Autodesk Inventor part; units mm, degrees
ref_plane "YZ Plane" through (0, 0, 0) normal (1, 0, 0) x (0, 1, 0)
ref_plane "XZ Plane" through (0, 0, 0) normal (0, 1, 0) x (-1, 0, 0)
ref_plane "XY Plane" through (0, 0, 0) normal (0, 0, 1) x (1, 0, 0)
sketch "Boceto1" plane through (0, 0, 0) normal (0, 1, 0) x (-1, 0, 0)
  circle A0 centre (0, 0) radius 20
  circle A1 centre (0, 0) radius 30
  line L0 (0, 0) -> (0, 60)
  line L1 (0, 60) -> (5, 60)
  line L2 (5, 60) -> (-5, 60)
  line L3 (-5, 60) -> (-5, 0)
  line L4 (-5, 0) -> (5, 0)
  line L5 (5, 0) -> (5, 60)
  line L6 (0, 60) -> (30, 60)
  line L7 (30, 60) -> (-30, 60)
  line L8 (-30, 60) -> (-30, 75)
  line L9 (-30, 75) -> (30, 75)
  line L10 (30, 75) -> (30, 60)
  point P0 (-5, 29.5804)
  point P1 (5, 29.5804)
  dimension "d0" = 40
  dimension "d1" = 60
  dimension "d2" = 60
  dimension "d3" = 5
  dimension "d4" = 10
  dimension "d5" = 30
  dimension "d6" = 60
  dimension "d7" = 15
extrude "Extrusión1" add sketch "Boceto1" along normal blind 60
sketch "Boceto2" plane through (30, 0, 75) normal (1, 0, 0) x (0, 0, -1)
  line L0 (0, 60) -> (15, 60)
  line L1 (0, 60) -> (0, 15)
  line L2 (0, 0) -> (0, 60)
  line L3 (0, 15) -> (75, 15)
  line L4 (75, 15) -> (75, 30)
  line L5 (75, 30) -> (15, 30)
  line L6 (15, 0) -> (15, 60)
  point P0 (75, 0)
  point P1 (15, 15)
  dimension "d10" = 45
  dimension "d11" = 15
extrude "Extrusión2" add sketch "Boceto2" against normal blind 60 contours L5 L4 L3 L6
sketch "Boceto3" plane through (30, 0, 75) normal (1, 0, 0) x (0, 0, -1)
  line L0 (45.4196, 15) -> (15, 15)
  line L1 (15, 15) -> (0, 15)
  line L2 (0, 0) -> (0, 60)
  line L3 (45.4196, 0) -> (15, 0)
  line L4 (0, 15) -> (45.4196, 15)
  line L5 (45.4196, 15) -> (45.4196, 0)
  line L6 (45.4196, 0) -> (0, 0)
  line L7 (0, 0) -> (0, 15)
  point P0 (75, 0)
extrude "Extrusión3" cut sketch "Boceto3" against normal blind 60
sketch "Boceto4" plane through (-30, 60, 75) normal (0, 0, 1) x (1, 0, 0)
  line L0 (60, 0) -> (0, 0)
  line L1 (30, 0) -> (47.5, 0)
  line L2 (47.5, 0) -> (47.5, -15)
  line L3 (30, 0) -> (30, -5.3607)
  circle A0 centre (47.5, -15) radius 8
  circle A1 centre (12.5, -15) radius 8
  point P0 (30, -60)
  point P1 (35, 0)
  point P2 (25, 0)
  dimension "d16" = 17.5
  dimension "d17" = 15
  dimension "d18" = 16
extrude "Extrusión4" cut sketch "Boceto4" against normal blind 15
sketch "Boceto5" plane through (0, 60, 0) normal (0, 1, 0) x (1, 0, 0)
  circle A0 centre (0, 0) radius 20
  dimension "d21" = 40
extrude "Extrusión5" cut sketch "Boceto5" against normal blind 60
sketch "Boceto6" plane through (0, 0, 0) normal (0, -1, 0) x (1, 0, 0)
  line L0 (0, 0) -> (0, -75)
  circle A0 centre (0, -75) radius 10
  circle A1 centre (0, -75) radius 23
  line L1 (0, -75) -> (23, -75)
  arc A2 (-5, 29.5804) -> (5, 29.5804) centre (0, 0) ccw
  line L2 (23, -19.2614) -> (23, -75)
  line L3 (-23, -19.2614) -> (-23, -75)
  dimension "d24" = 75
  dimension "d25" = 20
  dimension "d26" = 46
extrude "Extrusión6" add sketch "Boceto6" against normal blind 15 contours A2 L2 A1 L0 | L0 A1 L3 A2 | A1 L1 A0 L0 | L0 A0 L1 A1
sketch "Boceto7" plane through (0, 60, 0) normal (0, 1, 0) x (1, 0, 0)
  arc A0 (5, -29.5804) -> (-5, -29.5804) centre (0, 0) ccw
  line L0 (0, 30) -> (0, 55)
  line L1 (0, 55) -> (5, 55)
  line L2 (5, 29.5804) -> (5, 55)
  line L3 (0, 55) -> (-5, 55)
  line L4 (-5, 29.5804) -> (-5, 55)
  arc A1 (5, 29.5804) -> (-5, 29.5804) centre (0, 0) ccw
  dimension "d29" = 25
  dimension "d30" = 5
extrude "Extrusión7" add sketch "Boceto7" against normal blind 45
sketch "Boceto8" plane through (-5, 60, -55) normal (-1, 0, 0) x (0, 0, 1)
  line L0 (0, 0) -> (0, -45)
  line L1 (84.5804, 0) -> (25.4196, 0)
  line L2 (0, -45) -> (25.4196, 0)
  line L3 (35.7386, -45) -> (25.4196, -45)
  line L4 (25.4196, 0) -> (25.4196, -45)
  line L5 (25.4196, -45) -> (0, -45)
  line L6 (0, -45) -> (0, 0)
  line L7 (25.4196, 0) -> (0, 0)
  point P0 (55, -60)
extrude "Extrusión8" cut sketch "Boceto8" against normal blind 45 contours L7 L2 L0
Geometry check sheet. Reference: the model listing, model coordinates, mm. A direction names the side the tool comes from. Round coordinates to 2 decimals unless told otherwise and drop trailing zeros. Loops run counter-clockwise (first coordinate to the right, second up) from the corner with the lowest first, then second, coordinate; pieces in that order, holes last. Notation, with made-up numbers: (74.25, 33.25) -> (85.25, 33.25) arc R26 ccw to (85.25, 65.25) -> close; hole circle Ø7 at (26, 38). An arc over 180 degrees is marked (long way). Use a Markdown table: item, result.
(1) Scan lines: probe 1 along X at (y, z) = (5, -75); probe 2 along X at (y, z) = (42, 0); probe 3 along Z at (x, y) = (-14, 55). Record each from-to range of solid material in increasing order.
Calculated:
| item | result |
|---|---|
| probe 1 | -23 to -10, 10 to 23 |
| probe 2 | -30 to -20, 20 to 30 |
| probe 3 | -26.53 to -14.28, 14.28 to 26.53, 60 to 75 |
(2) Mould release check, pull along Z, two halves, no side actions. Record for faces 1 (the flat face through (0, 8, 29.58)), 2 (the cylindrical face through (5.38, 7.4, -66.57)), 3 (the cylindrical face through (11.6, 50.4, 67.6)): released by +Z, released by -Z, zero draft, split by the parting line, or undercut.
Calculated:
| item | result |
|---|---|
| face 1 | released by +Z |
| face 2 | undercut |
| face 3 | zero draft |
(3) Sectioned sample at B-B (x = 0). Enter the section's corners in (y, z).
Calculated:
| item | result |
|---|---|
| outline | (0, -98) -> (15, -98) -> (15, -85) -> (0, -85) -> close; (0, -65) -> (15, -65) -> (15, -55) -> (60, -29.58) -> (60, -20) -> (0, -20) -> close; (0, 20) -> (60, 20) -> (60, 75) -> (15, 75) -> (15, 29.58) -> (0, 29.58) -> close |
(4) Sectioned sample at D-D (z = -10). Enter the section's corners in (x, y).
Calculated:
| item | result |
|---|---|
| outline | (-28.28, 0) -> (-17.32, 0) -> (-17.32, 60) -> (-28.28, 60) -> close; (17.32, 0) -> (28.28, 0) -> (28.28, 60) -> (17.32, 60) -> close |
(5) Sectioned sample at A-A (y = 45). Enter the section's corners in (x, z).
Calculated:
| item | result |
|---|---|
| outline | (-30, 60) -> (-25.5, 60) -> (-25.5, 75) -> (-30, 75) -> close; (-9.5, 60) -> (-5, 60) -> (-5, 29.58) arc R30 ccw to (-5, -29.58) -> (-5, -38.05) -> (5, -38.05) -> (5, -29.58) arc R30 ccw to (5, 29.58) -> (5, 60) -> (9.5, 60) -> (9.5, 75) -> (-9.5, 75) -> close; (25.5, 60) -> (30, 60) -> (30, 75) -> (25.5, 75) -> close; hole circle Ø40 at (0, 0) |
(6) Go/stop test with flat-tipped pins: P1, Ø12, axis at x = -21, y = 16, coming from the -Z side; P2, Ø3, axis at x = -9.5, y = 16, coming from the -Z side; P3, Ø11, axis at x = 2, y = 7.5, coming from the +Z side; P4, Ø16, axis at x = 0, z = -75, coming from the +Y side. Record where each tip stops, or that it passes through.
Calculated:
| item | result |
|---|---|
| P1 | z = -92.36 |
| P2 | z = -96.42 |
| P3 | z = 29.58 |
| P4 | through |
(7) Sectioned sample at C-C (y = 12). Enter the section's corners in (x, z), then the cut area to 3 significant figures.
Calculated:
| item | result |
|---|---|
| outline | (-23, -75) arc R23 ccw to (23, -75) -> (23, -19.26) arc R30 ccw to (5, 29.58) -> (-5, 29.58) arc R30 ccw to (-23, -19.26) -> close; hole circle Ø40 at (0, 0); hole circle Ø20 at (0, -75) |
| area | 4,310 mm² |
(8) Set-up check for faces 4 (the cylindrical face through (-29.994, 36.247, 0.589)), 5 (the flat face through (-5, 45, 45)), 6 (the flat face through (18, 30, 43)), 7 (the cylindrical face through (29.994, 29.58, -0.589)): record each of +Z, -Z, +X, -X, +Y, -Y from which the full face is reachable in a straight line by a thin tool's end or side.
Calculated:
| item | result |
|---|---|
| face 4 | -X |
| face 5 | -X, +Y |
| face 6 | +X, +Y |
| face 7 | +X |
